Work out the finished part from the listing and answer in its coordinate system (mm). Give positions to 0.01 mm unless a question says otherwise; leave off trailing zeros. Loops run counter-clockwise (first coordinate to the right, second up) from the corner with the lowest first, then second, coordinate; pieces in that order, holes last. Notation, with made-up numbers: (83, 28.5) - (142, 28.5) arc R20 ccw to (142, 34.5) - close; hole circle Ø6 at (-2, 68.25). An arc over 180 degrees is marked (long way). Use CSV: the item, a comma, the result in double quotes.
from build123d import *

# Parameters (mm, degrees)
BOSS_EXTRUDE1_DEPTH = 140


with BuildPart() as part:
    # Sketch4 → Boss-Extrude1 (new body)
    with BuildSketch(Plane(origin=(0, 0, 0), x_dir=(1, 0, 0), z_dir=(0, 1, 0))):
        with BuildLine():
            ThreePointArc((10, 0), (0, -10), (-10, 0))
            Line((-10, 0), (-20, 0))
            Line((-20, 0), (-20, -25))
            Line((-20, -25), (20, -25))
            Line((20, -25), (20, 0))
            Line((20, 0), (10, 0))
        make_face()
    extrude(amount=-BOSS_EXTRUDE1_DEPTH)


solid = part.part
Item 1: Find the intervals of material crossed by line 1 (Z direction, x = 0.5, y = -41); line 2 (X direction, y = -60, z = 6.5); line 3 (X direction, y = -89, z = 6.75), in increasing order.
Determined:
line 1,"z = 9.99 to 25"
line 2,"x = -20 to -7.6, 7.6 to 20"
line 3,"x = -20 to -7.38, 7.38 to 20"
Item 2: A cutting plane is placed at D-D on x = -6. Determine the outline of the cut face in (y, z), and give its area (3 significant figures).
Determined:
outline,"(-140, 8) - (0, 8) - (0, 25) - (-140, 25) - close"
area,"2,380 mm²"
Item 3: A cutting plane is placed at A-A on z = 6. Determine the outline of the cut face in (x, y).
Determined:
outline,"(-20, -140) - (-8, -140) - (-8, 0) - (-20, 0) - close; (8, -140) - (20, -140) - (20, 0) - (8, 0) - close"
Item 4: A cutting plane is placed at B-B on y = -101. Determine the outline of the cut face in (x, z).
Determined:
outline,"(-20, 0) - (-10, 0) arc R10 cw to (10, 0) - (20, 0) - (20, 25) - (-20, 25) - close"
Item 5: A cutting plane is placed at C-C on x = 0. Determine the outline of the cut face in (y, z), and give its area (3 significant figures).
Determined:
outline,"(-140, 10) - (0, 10) - (0, 25) - (-140, 25) - close"
area,"2,100 mm²"
Item 6: Given P1, Ø12, axis at x = -5.5, y = -62, coming from the -Z side; P2, Ø2, axis at x = -3, y = -73, coming from the -Z side, each flat-ended and moving along its own axis, determine where each tip first touches the part or whether it passes through.
Determined:
P1,"stops at z = 0"
P2,"stops at z = 9.17"
Item 7: The mould has two halves that part along X. Classify faces 1 (the flat face through (20, -69, 13)), 2 (the cylindrical face through (0, -69, 10)), 3 (the flat face through (0, -69, 25)): pulls with the +X half, pulls with the -X half, needs draft (parallel to the pull), parting line crosses it, or undercut.
Determined:
face 1,"pulls with the +X half"
face 2,"undercut"
face 3,"needs draft"
